Verification items for the finished model (mm, model axes). Face numbers are marked on the shaded views. A direction names the side the tool comes from. Give positions to 0.01 mm unless a question says otherwise; leave off trailing zeros. Order: outer loops, then holes, each group sorted by start corner. A loop starts at its lowest first (then second) coordinate and runs counter-clockwise, first axis right, second up. Notation, with made-up numbers: (-26, 24.5) - (23, 24.5) arc R17 ccw to (23, 47.5) - close; hole circle Ø7 at (-7, -6). An arc over 180 degrees is marked (long way). Answer as a JSON object with one key per item and string values. Group by question number.
(1) Thickness scan on line 1 (X direction, y = 40, z = -50); line 2 (Z direction, x = -33.5, y = 4); line 3 (Y direction, x = -23, z = -26). Record the ranges inside material, lowest first.
(2) Section check D-D (z = -75.5). Record the boundary of the cut face in (x, y), then the cut area to 4 significant figures.
(3) Mould release check, pull along X, two halves, no side actions. Record for the marked faces 1, 2, 3 and 4: +X half, -X half, draft (parallel to the pull), parting line (faces both ways), or undercut.
(4) Section check C-C (x = -26). Record the boundary of the cut face in (y, z), then the cut area to 3 significant figures.
(5) Section check B-B (x = -96). Record the boundary of the cut face in (y, z).
(6) Depth check by flat-ended pin: pin 1 Ø0.9 at (x, z) = (-111, -53) entering from +Y; pin 2 Ø0.8 at (x, z) = (-70.5, -0.5) entering from +Y; pin 3 Ø8 at (x, z) = (-21.5, -35) entering from +Y. Enter the tip coordinate at first touch or a pass-through.
(7) Access from +Z, -Z, +X, -X, +Y, -Y to the whole of each face (thin tool, end or side, straight path). Record for the marked faces 5 and 6.
(8) Section check A-A (y = 14). Record the boundary of the cut face in (x, z), then the cut area to 3 significant figures.
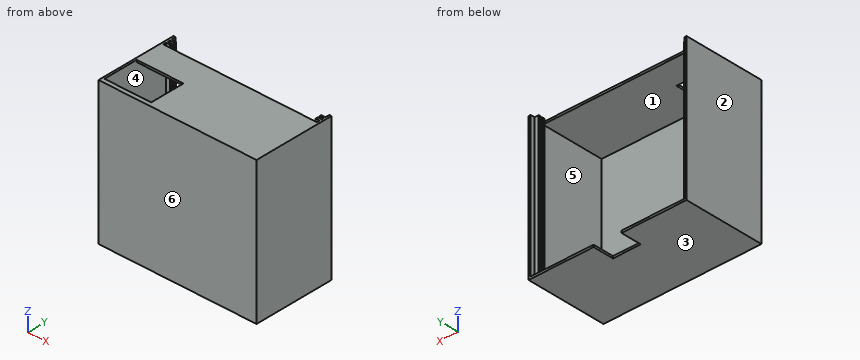
Autodesk Inventor part; units mm, degrees
ref_plane "YZ Plane" through (0, 0, 0) normal (1, 0, 0) x (0, 1, 0)
ref_plane "XZ Plane" through (0, 0, 0) normal (0, 1, 0) x (-1, 0, 0)
ref_plane "XY Plane" through (0, 0, 0) normal (0, 0, 1) x (1, 0, 0)
sketch "Sketch1" plane through (0, 0, 0) normal (0, 1, 0) x (-1, 0, 0)
  line L0 (0, 0) -> (113.5, 0)
  line L1 (113.5, 0) -> (113.5, -103)
  line L2 (113.5, -103) -> (0, -103)
  line L3 (0, -103) -> (0, 0)
  dimension "d0" = 113.5
  dimension "d1" = 103
extrude "Extrusion1" add sketch "Sketch1" along normal blind 3
sketch "Sketch2" plane through (0, 3, 0) normal (0, 1, 0) x (1, 0, 0)
  line L0 (0, 0) -> (0, 103)
  line L1 (-113.5, 0) -> (0, 0)
  line L2 (0, 103) -> (-113.5, 103)
  line L3 (-113.5, 103) -> (-113.5, 0)
  line L4 (-112, 51.5) -> (-112, 0)
  line L5 (-56.75, 101.5) -> (-112, 101.5)
  line L6 (-112, 101.5) -> (-1.5, 101.5)
  line L7 (-1.5, 101.5) -> (-1.5, 0)
  line L8 (-112, 0) -> (-112, 101.5)
extrude "Extrusion2" add sketch "Sketch2" along normal blind 55 contours L1 L7 L6 L5 L8 L4 L3 L2 L0
sketch "Sketch3" plane through (-112, 3, -101.5) normal (0, 0, 1) x (1, 0, 0)
  point P0 (112, -3)
sketch "Sketch4" plane through (-112, 3, -101.5) normal (0, 0, 1) x (1, 0, 0)
  line L0 (0, 55) -> (110.5, 55)
  line L1 (65.25, 40) -> (45.25, 40)
  line L2 (45.25, 40) -> (45.25, 55)
  line L3 (65.25, 40) -> (65.25, 55)
  line L4 (45.25, 55) -> (65.25, 55)
  point P0 (112, -3)
  dimension "d11" = 20
extrude "Extrusion3" cut sketch "Sketch4" against normal through all
sketch "Sketch5" plane through (-112, 3, 0) normal (1, 0, 0) x (0, 0, -1)
  line L0 (0, 55) -> (101.5, 55)
  line L1 (0, 0) -> (0, 55)
  line L2 (0, 52.0001) -> (101.5, 52.0001)
  line L3 (101.5, 0) -> (101.5, 55)
  line L4 (101.5, 52.0001) -> (101.5, 50.5001)
  line L5 (101.5, 50.5001) -> (0, 50.5001)
  line L6 (0, 52.0001) -> (0, 50.5001)
  line L7 (0, 49.0001) -> (101.5, 49.0001)
  line L8 (101.5, 49.0001) -> (101.5, 47.5001)
  line L9 (101.5, 47.5001) -> (0, 47.5001)
  line L10 (0, -3) -> (0, 55)
  line L11 (0, 49.0001) -> (0, 47.5001)
  dimension "d14" = 1.5
  dimension "d15" = 1.5
  dimension "d16" = 1.5
extrude "Extrusion4" add sketch "Sketch5" along normal blind 3 contours L2 L3 L5 L1 | L7 L3 L9 L1
sketch "Sketch6" plane through (-1.5, 3, -101.5) normal (-1, 0, 0) x (0, 0, 1)
  line L0 (0, 55) -> (101.5, 55)
  line L1 (0, 0) -> (0, 55)
  line L2 (0, 52) -> (101.5, 52)
  line L3 (101.5, 0) -> (101.5, 55)
  line L4 (101.5, 52) -> (101.5, 50.5)
  line L5 (101.5, 50.5) -> (0, 50.5)
  line L6 (0, 50.5) -> (0, 52)
  line L7 (101.5, 49) -> (0, 49)
  line L8 (0, 49) -> (0, 47.5)
  line L9 (0, 47.5) -> (101.5, 47.5)
  line L10 (101.5, -3) -> (101.5, 55)
  line L11 (101.5, 49) -> (101.5, 47.5)
  dimension "d20" = 1.5
  dimension "d21" = 1.5
  dimension "d22" = 1.5
extrude "Extrusion5" add sketch "Sketch6" along normal blind 3 contours L2 L3 L5 L1 | L7 L3 L9 L1
sketch "Sketch8" plane through (-1.5, 3, -101.5) normal (-1, 0, 0) x (0, 0, 1)
  line L0 (101.5, 0) -> (101.5, 47.5)
  line L1 (101.5, 45.3848) -> (101.5, 43.8848)
  line L2 (101.5, 45.3848) -> (100, 45.3848)
  line L3 (100, 45.3848) -> (100, 24.9998)
  line L4 (100, 24.9998) -> (101.5, 24.9998)
  line L5 (101.5, -3) -> (101.5, 55)
  dimension "d27" = 1.5
  dimension "d28" = 1.5
  dimension "d29" = 20.385
extrude "Extrusion6" add sketch "Sketch8" along normal up to surface (110.5 mm away)
sketch "Sketch10" plane through (-112, 27.9998, -1.5) normal (0, -1, 0) x (1, 0, 0)
  line L0 (110.5, 1.5) -> (0, 1.5)
  line L1 (33.533, 1.5) -> (33.533, 0)
  line L2 (110.5, 0) -> (0, 0)
  line L3 (33.4948, 1.5) -> (110.5, 1.5)
  line L4 (110.5, 1.5) -> (110.5, 0)
  line L5 (110.5, 1.5) -> (110.5, 0)
  line L6 (110.5, 0) -> (33.533, 0)
  point P0 (112, 1.5)
extrude "Extrusion7" add sketch "Sketch10" along normal up to surface (24.9998 mm away)
properties part number "casingN"
Solutions:
{
 "1": {"line 1": "x = -113.5 to -112, -1.5 to 0", "line 2": "z = -103 to -101.5, -1.5 to 0", "line 3": "y = 0 to 3"},
 "2": {"outline": "(-113.5, 0) - (0, 0) - (0, 58) - (-1.5, 58) - (-1.5, 55) - (-4.5, 55) - (-4.5, 53.5) - (-1.5, 53.5) - (-1.5, 52) - (-4.5, 52) - (-4.5, 50.5) - (-1.5, 50.5) - (-1.5, 3) - (-112, 3) - (-112, 50.5) - (-109, 50.5) - (-109, 52) - (-112, 52) - (-112, 53.5) - (-109, 53.5) - (-109, 55) - (-112, 55) - (-112, 58) - (-113.5, 58) - close", "area": "523.5 mm2"},
 "3": {"face 1": "undercut", "face 2": "-X half", "face 3": "draft", "face 4": "undercut"},
 "4": {"outline": "(0, -103) - (58, -103) - (58, -101.5) - (3, -101.5) - (3, -1.5) - (48.38, -1.5) - (48.38, 0) - (0, 0) - close", "area": "460 mm2"},
 "5": {"outline": "(0, -103) - (58, -103) - (58, -101.5) - (3, -101.5) - (3, 0) - (0, 0) - close; (28, -1.5) - (48.38, -1.5) - (48.38, 0) - (28, 0) - close"},
 "6": {"pin 1": "stops at y = 55", "pin 2": "stops at y = 48.38", "pin 3": "stops at y = 3"},
 "7": {"face 5": "none", "face 6": "+Z, -Z, +X, -X, -Y"},
 "8": {"outline": "(-113.5, -103) - (0, -103) - (0, 0) - (-78.47, 0) - (-78.47, -1.5) - (-1.5, -1.5) - (-1.5, -101.5) - (-112, -101.5) - (-112, 0) - (-113.5, 0) - close", "area": "590 mm2"}
}
